```python
from build123d import *

# Parameters (mm, degrees)
BOSS_EXTRUDE1_DEPTH       = 20
SKETCH2_W                 = 20
SKETCH2_H                 = 40
CUT_EXTRUDE1_DEPTH        = 142.509716981
SHELL1_T                  = -2
SHELL1_THICKNESS_2_FACE_W = 20
SHELL1_THICKNESS_2_FACE_H = 18
SHELL1_THICKNESS_2_DEPTH  = 3
SHELL1_THICKNESS_3_FACE_W = 18
SHELL1_THICKNESS_3_FACE_H = 20
SHELL1_THICKNESS_3_DEPTH  = 3
CUT_EXTRUDE14_REACH       = 110.167
SKETCH34_R                = 2.5
SKETCH3_W                 = 2.5
SKETCH3_H                 = 10
BOSS_EXTRUDE2_DEPTH       = 5
FILLET2_R                 = 5
CUT_EXTRUDE3_REACH        = 149.838
SKETCH6_R                 = 1.5
SKETCH21_R                = 2.5
SKETCH21_R_2              = 1.5
BOSS_EXTRUDE10_DEPTH      = 2.5
BOSS_EXTRUDE10_DRAFT      = 3
MIRROR7_COPY_1_SKETCH_R   = 2.5
MIRROR7_COPY_1_SKETCH_R_2 = 1.5
MIRROR7_COPY_1_DEPTH      = 2.5
MIRROR7_COPY_1_DRAFT      = 3
SKETCH26_W                = 5
SKETCH26_H                = 10
CUT_EXTRUDE8_DEPTH        = 2
SKETCH7_W                 = 2.5
SKETCH7_H                 = 10
BOSS_EXTRUDE4_DEPTH       = 5
FILLET4_R                 = 5
SKETCH22_R                = 2.5
BOSS_EXTRUDE11_DEPTH      = 2.5
BOSS_EXTRUDE11_TAPER      = 3
SKETCH23_R                = 1.5
CUT_EXTRUDE7_DEPTH        = 10
SKETCH27_W                = 5
SKETCH27_H                = 10
CUT_EXTRUDE9_DEPTH        = 2
SKETCH10_W                = 2.5
SKETCH10_H                = 10
BOSS_EXTRUDE6_DEPTH       = 5
FILLET6_R                 = 5
SKETCH28_R                = 2.5
BOSS_EXTRUDE12_DEPTH      = 2.5
BOSS_EXTRUDE12_TAPER      = 3
SKETCH29_R                = 1.5
CUT_EXTRUDE10_DEPTH       = 10
SKETCH30_W                = 5
SKETCH30_H                = 10
CUT_EXTRUDE11_DEPTH       = 2
SKETCH13_W                = 2.5
SKETCH13_H                = 10
BOSS_EXTRUDE8_DEPTH       = 5
FILLET8_R                 = 5
SKETCH31_R                = 2.5
BOSS_EXTRUDE13_DEPTH      = 2.5
BOSS_EXTRUDE13_TAPER      = 3
SKETCH32_R                = 1.5
CUT_EXTRUDE12_DEPTH       = 10
SKETCH33_W                = 5
SKETCH33_H                = 10
CUT_EXTRUDE13_DEPTH       = 2


with BuildPart() as part:
    # Sketch1 → Boss-Extrude1 (new body)
    with BuildSketch(Plane.XY):
        Polygon((58, 114), (58, 115), (80, 115), (80, 20), (60, 0), (0, 0), (-10, 25), (-10, 105), (11, 105), (11, 110), (12, 110), (34, 110), (34, 115), (35, 115), (57, 115), (57, 114), align=None)
        Polygon((80, 14.004150764), (60, 0), (80, 20), align=None)
    extrude(amount=BOSS_EXTRUDE1_DEPTH)

    # Sketch2 → Cut-Extrude1 (cut, through all)
    with BuildSketch(Plane.XY.offset(20)):
        with Locations((70, 45)):
            Rectangle(SKETCH2_W, SKETCH2_H)
    extrude(amount=-CUT_EXTRUDE1_DEPTH, mode=Mode.SUBTRACT)

    # Shell1
    shell1_openings = [part.faces().sort_by_distance(p)[0] for p in [
        (32.82341614, 58.185068385, 20),
    ]]
    offset(amount=SHELL1_T, openings=shell1_openings, kind=Kind.INTERSECTION)

    # Shell1 thickness 2 face (on inner face of the shell) → Shell1 thickness 2 (add)
    with BuildSketch(Plane(origin=(68, 23, 11), x_dir=(1, 0, 0), z_dir=(0, 1, 0))):
        Rectangle(SHELL1_THICKNESS_2_FACE_W, SHELL1_THICKNESS_2_FACE_H)
    extrude(amount=-SHELL1_THICKNESS_2_DEPTH)

    # Shell1 thickness 3 face (on inner face of the shell) → Shell1 thickness 3 (add)
    with BuildSketch(Plane(origin=(68, 67, 11), x_dir=(0, 0, -1), z_dir=(0, -1, 0))):
        Rectangle(SHELL1_THICKNESS_3_FACE_W, SHELL1_THICKNESS_3_FACE_H)
    extrude(amount=-SHELL1_THICKNESS_3_DEPTH)

    # Cut-Extrude14: up to this face of the body (flat: up to its plane)
    cut_extrude14_end = Plane(part.part.faces().sort_by_distance((68, 20, 11))[0])
    # Sketch34 → Cut-Extrude14 (cut, up to the picked face)
    with BuildSketch(Plane(origin=(0, 70, 0), x_dir=(1, 0, 0), z_dir=(0, 1, 0)), mode=Mode.PRIVATE) as cut_extrude14_sk1:
        with Locations(Location((70, -11, 0), (0, 0, 270))):
            Circle(SKETCH34_R)
    cut_extrude14_tool1 = split(extrude(cut_extrude14_sk1.sketch, amount=-CUT_EXTRUDE14_REACH, mode=Mode.PRIVATE), bisect_by=cut_extrude14_end, keep=Keep.BOTH, mode=Mode.PRIVATE)
    add(cut_extrude14_tool1.solids().sort_by(Axis((70, 70, 11), (0, -1, 0)))[0], mode=Mode.SUBTRACT)

    # Sketch3 → Boss-Extrude2 (add)
    with BuildSketch(Plane(origin=(0, 115, 0), x_dir=(1, 0, 0), z_dir=(0, 1, 0))):
        with Locations((65.25, -10)):
            Rectangle(SKETCH3_W, SKETCH3_H)
        with Locations((72.75, -10)):
            Rectangle(SKETCH3_W, SKETCH3_H)
    extrude(amount=BOSS_EXTRUDE2_DEPTH)

    # Fillet2
    fillet2_edges = [part.edges().sort_by_distance(p)[0] for p in [
        (65.25, 120, 5),
        (65.25, 120, 15),
        (72.75, 120, 5),
        (72.75, 120, 15),
    ]]
    fillet(fillet2_edges, radius=FILLET2_R - 0.0001)  # a hair under: the kernel refuses the full size

    # Cut-Extrude3: up to this face of the body (flat: up to its plane)
    cut_extrude3_end = Plane(part.part.faces().sort_by_distance((64, 117.122079053, 10))[0])
    # Sketch6 → Cut-Extrude3 (cut, up to the picked face)
    with BuildSketch(Plane(origin=(74, 0, 0), x_dir=(0, 0, -1), z_dir=(1, 0, 0)), mode=Mode.PRIVATE) as cut_extrude3_sk1:
        with Locations((-10, 117.5)):
            Circle(SKETCH6_R)
    cut_extrude3_tool1 = split(extrude(cut_extrude3_sk1.sketch, amount=-CUT_EXTRUDE3_REACH, mode=Mode.PRIVATE), bisect_by=cut_extrude3_end, keep=Keep.BOTH, mode=Mode.PRIVATE)
    add(cut_extrude3_tool1.solids().sort_by(Axis((74, 117.5, 10), (-1, 0, 0)))[0], mode=Mode.SUBTRACT)


with BuildPart() as boss_extrude10_tool:
    # Sketch21 → Boss-Extrude10 (with draft: the straight prism first)
    with BuildSketch(Plane(origin=(66.5, 0, 0), x_dir=(0, 0, -1), z_dir=(1, 0, 0))):
        with Locations((-10, 117.5)):
            Circle(SKETCH21_R)
        with Locations((-10, 117.5)):
            Circle(SKETCH21_R_2, mode=Mode.SUBTRACT)
    extrude(amount=BOSS_EXTRUDE10_DEPTH)
    # Boss-Extrude10: the draft: its side faces are tilted about the plane it starts from
    boss_extrude10_sides = [boss_extrude10_tool.faces().sort_by_distance(p)[0] for p in [
        (67.75, 117.5, 12.5),
        (67.75, 117.5, 11.5),
    ]]
    draft(boss_extrude10_sides, Plane(origin=(66.5, 0, 0), x_dir=(0, 0, -1), z_dir=(1, 0, 0)), BOSS_EXTRUDE10_DRAFT)


with BuildPart() as part_1:
    add(part.part)

    # Boss-Extrude10: add boss_extrude10_tool
    add(boss_extrude10_tool.part)


with BuildPart() as mirror7_copy_1_tool:
    # Mirror7 copy 1 sketch → Mirror7 copy 1 (with draft: the straight prism first)
    with BuildSketch(Plane(origin=(71.5, 0, 0), x_dir=(0, 0, -1), z_dir=(-1, 0, 0))):
        with Locations((-10, -117.5)):
            Circle(MIRROR7_COPY_1_SKETCH_R)
        with Locations((-10, -117.5)):
            Circle(MIRROR7_COPY_1_SKETCH_R_2, mode=Mode.SUBTRACT)
    extrude(amount=MIRROR7_COPY_1_DEPTH)
    # Mirror7 copy 1: the draft: its side faces are tilted about the plane it starts from
    mirror7_copy_1_sides = [mirror7_copy_1_tool.faces().sort_by_distance(p)[0] for p in [
        (70.25, 117.5, 12.5),
        (70.25, 117.5, 11.5),
    ]]
    draft(mirror7_copy_1_sides, Plane(origin=(71.5, 0, 0), x_dir=(0, 0, -1), z_dir=(-1, 0, 0)), MIRROR7_COPY_1_DRAFT)


with BuildPart() as part_2:
    add(part_1.part)

    # Mirror7 copy 1: add mirror7_copy_1_tool
    add(mirror7_copy_1_tool.part)

    # Sketch26 → Cut-Extrude8 (cut)
    with BuildSketch(Plane(origin=(0, 115, 0), x_dir=(1, 0, 0), z_dir=(0, 1, 0))):
        with Locations((69, -10)):
            Rectangle(SKETCH26_W, SKETCH26_H)
    extrude(amount=-CUT_EXTRUDE8_DEPTH, mode=Mode.SUBTRACT)

    # Sketch7 → Boss-Extrude4 (add)
    with BuildSketch(Plane(origin=(0, 115, 0), x_dir=(1, 0, 0), z_dir=(0, 1, 0))):
        with Locations((41.25, -10)):
            Rectangle(SKETCH7_W, SKETCH7_H)
        with Locations((48.75, -10)):
            Rectangle(SKETCH7_W, SKETCH7_H)
    extrude(amount=BOSS_EXTRUDE4_DEPTH)

    # Fillet4
    fillet4_edges = [part_2.edges().sort_by_distance(p)[0] for p in [
        (41.25, 120, 5),
        (41.25, 120, 15),
        (48.75, 120, 5),
        (48.75, 120, 15),
    ]]
    fillet(fillet4_edges, radius=FILLET4_R - 0.0001)  # a hair under: the kernel refuses the full size

    # Sketch22 → Boss-Extrude11 (add)
    with BuildSketch(Plane(origin=(42.5, 0, 0), x_dir=(0, 0, -1), z_dir=(1, 0, 0))):
        with Locations((-10, 117.5)):
            Circle(SKETCH22_R)
    boss_extrude11 = extrude(amount=BOSS_EXTRUDE11_DEPTH, taper=BOSS_EXTRUDE11_TAPER)

    # Mirror8: Boss-Extrude11 across plane
    add(boss_extrude11.mirror(Plane(origin=(45, 117.5, 10), x_dir=(0, 0, 1), z_dir=(1, 0, 0))))

    # Sketch23 → Cut-Extrude7 (cut)
    with BuildSketch(Plane(origin=(50, 0, 0), x_dir=(0, 0, -1), z_dir=(1, 0, 0))):
        with Locations((-10, 117.5)):
            Circle(SKETCH23_R)
    extrude(amount=-CUT_EXTRUDE7_DEPTH, mode=Mode.SUBTRACT)

    # Sketch27 → Cut-Extrude9 (cut)
    with BuildSketch(Plane(origin=(0, 115, 0), x_dir=(1, 0, 0), z_dir=(0, 1, 0))):
        with Locations((45, -10)):
            Rectangle(SKETCH27_W, SKETCH27_H)
    extrude(amount=-CUT_EXTRUDE9_DEPTH, mode=Mode.SUBTRACT)

    # Sketch10 → Boss-Extrude6 (add)
    with BuildSketch(Plane(origin=(0, 110, 0), x_dir=(1, 0, 0), z_dir=(0, 1, 0))):
        with Locations((19.25, -10)):
            Rectangle(SKETCH10_W, SKETCH10_H)
        with Locations((26.75, -10)):
            Rectangle(SKETCH10_W, SKETCH10_H)
    extrude(amount=BOSS_EXTRUDE6_DEPTH)

    # Fillet6
    fillet6_edges = [part_2.edges().sort_by_distance(p)[0] for p in [
        (19.25, 115, 15),
        (19.25, 115, 5),
        (26.75, 115, 5),
        (26.75, 115, 15),
    ]]
    fillet(fillet6_edges, radius=FILLET6_R - 0.0001)  # a hair under: the kernel refuses the full size

    # Sketch28 → Boss-Extrude12 (add)
    with BuildSketch(Plane(origin=(20.5, 0, 0), x_dir=(0, 0, -1), z_dir=(1, 0, 0))):
        with Locations((-10, 112.5)):
            Circle(SKETCH28_R)
    boss_extrude12 = extrude(amount=BOSS_EXTRUDE12_DEPTH, taper=BOSS_EXTRUDE12_TAPER)

    # Mirror9: Boss-Extrude12 across plane
    add(boss_extrude12.mirror(Plane(origin=(23, 112.5, 10), x_dir=(0, 0, 1), z_dir=(1, 0, 0))))

    # Sketch29 → Cut-Extrude10 (cut)
    with BuildSketch(Plane(origin=(28, 0, 0), x_dir=(0, 0, -1), z_dir=(1, 0, 0))):
        with Locations((-10, 112.5)):
            Circle(SKETCH29_R)
    extrude(amount=-CUT_EXTRUDE10_DEPTH, mode=Mode.SUBTRACT)

    # Sketch30 → Cut-Extrude11 (cut)
    with BuildSketch(Plane(origin=(0, 110, 0), x_dir=(1, 0, 0), z_dir=(0, 1, 0))):
        with Locations((23, -10)):
            Rectangle(SKETCH30_W, SKETCH30_H)
    extrude(amount=-CUT_EXTRUDE11_DEPTH, mode=Mode.SUBTRACT)

    # Sketch13 → Boss-Extrude8 (add)
    with BuildSketch(Plane(origin=(0, 105, 0), x_dir=(1, 0, 0), z_dir=(0, 1, 0))):
        with Locations((-2.75, -10)):
            Rectangle(SKETCH13_W, SKETCH13_H)
        with Locations((4.75, -10)):
            Rectangle(SKETCH13_W, SKETCH13_H)
    extrude(amount=BOSS_EXTRUDE8_DEPTH)

    # Fillet8
    fillet8_edges = [part_2.edges().sort_by_distance(p)[0] for p in [
        (-2.75, 110, 15),
        (-2.75, 110, 5),
        (4.75, 110, 5),
        (4.75, 110, 15),
    ]]
    fillet(fillet8_edges, radius=FILLET8_R - 0.0001)  # a hair under: the kernel refuses the full size

    # Sketch31 → Boss-Extrude13 (add)
    with BuildSketch(Plane(origin=(-1.5, 0, 0), x_dir=(0, 0, -1), z_dir=(1, 0, 0))):
        with Locations((-10, 107.5)):
            Circle(SKETCH31_R)
    boss_extrude13 = extrude(amount=BOSS_EXTRUDE13_DEPTH, taper=BOSS_EXTRUDE13_TAPER)

    # Mirror10: Boss-Extrude13 across plane
    add(boss_extrude13.mirror(Plane(origin=(1, 107.5, 10), x_dir=(0, 0, 1), z_dir=(1, 0, 0))))

    # Sketch32 → Cut-Extrude12 (cut)
    with BuildSketch(Plane(origin=(6, 0, 0), x_dir=(0, 0, -1), z_dir=(1, 0, 0))):
        with Locations((-10, 107.5)):
            Circle(SKETCH32_R)
    extrude(amount=-CUT_EXTRUDE12_DEPTH, mode=Mode.SUBTRACT)

    # Sketch33 → Cut-Extrude13 (cut)
    with BuildSketch(Plane(origin=(0, 105, 0), x_dir=(1, 0, 0), z_dir=(0, 1, 0))):
        with Locations((1, -10)):
            Rectangle(SKETCH33_W, SKETCH33_H)
    extrude(amount=-CUT_EXTRUDE13_DEPTH, mode=Mode.SUBTRACT)


solid = part_2.part
```
Verification items for the finished model (mm, model axes). A direction names the side the tool comes from. Round coordinates to 2 decimals unless told otherwise and drop trailing zeros. Write each loop counter-clockwise with the first axis right and the second up, starting at its lowest first coordinate (ties: lowest second). Pieces come first, ordered by that corner, then holes. Notation, with made-up numbers: (-10, 86.5) -> (4, 86.5) arc R36 cw to (4, 124.5) -> close; hole circle Ø8 at (1.5, -32.75). An arc over 180 degrees is marked (long way). Write each question's results on one line, items separated by ' | '.
Q1. Go/stop test with flat-tipped pins: pin 1 Ø2 at (y, z) = (113, 8.5) entering from -X; pin 2 Ø1.5 at (y, z) = (106, 2.5) entering from -X; pin 3 Ø1.5 at (y, z) = (117, 12.5) entering from +X. Record where each tip stops, or that it passes through.
Derived:
pin 1: stops at x = 18 | pin 2: stops at x = 11 | pin 3: stops at x = 74
Q2. Thickness scan on probe 1 along Y at (x, z) = (15, 6); probe 2 along Y at (x, z) = (44, 16.75); probe 3 along Y at (x, z) = (64, 18.25). Record the ranges inside material, lowest first.
Derived:
probe 1: y = 0 to 2, 108 to 110 | probe 2: y = 0 to 2, 113 to 115 | probe 3: y = 2.8 to 5.24, 20 to 25, 65 to 70, 113 to 115
Q3. Access from +Z, -Z, +X, -X, +Y, -Y to the whole of each face (thin tool, end or side, straight path). Record for faces 5 (the face through (2.232, 109.913, 10.317)), 6 (the face through (60, 45, 10)), 7 (the face through (1, 109, 10)), 8 (the face through (68, 20, 13)).
Derived:
face 5: none | face 6: +Z, -Z, +X | face 7: -X | face 8: +Z
Q4. Sectioned sample at B-B, the plane y = 117.5. Give the number of separate pieces and of enclosed holes in the cut face, and give its area (3 significant figures).
Derived:
separate pieces: 4 | enclosed holes: 0 | area: 74.6 mm²
Q5. Draft check along Y on faces 1 (the face through (41, 118, 6)), 2 (the face through (-4, 105.8, 10.1)), 3 (the face through (13, 105, 11)), 4 (the face through (27, 108, 11)). Enter one of: released by +Y, released by -Y, zero draft, split by the parting line, or undercut.
Derived:
face 1: released by +Y | face 2: zero draft | face 3: undercut | face 4: undercut
Q6. Sectioned sample at A-A, the plane x = 30. Record the boundary of the cut face in (y, z).
Derived:
outline: (0, 0) -> (110, 0) -> (110, 20) -> (108, 20) -> (108, 2) -> (2, 2) -> (2, 20) -> (0, 20) -> close
